Here's how the part is built. I have some questions about the finished solid (model axes, mm). Face numbers are marked on the shaded views. A direction names the side the tool comes from. Round coordinates to 2 decimals unless told otherwise and drop trailing zeros. Write each loop counter-clockwise with the first axis right and the second up, starting at its lowest first coordinate (ties: lowest second). Pieces come first, ordered by that corner, then holes. Notation, with made-up numbers: (21.25, 23) - (61.25, 23) arc R20 ccw to (61.25, 49) - close; hole circle Ø4 at (-6, -37). An arc over 180 degrees is marked (long way). Use one line per item in the form item = value. Start each with the question number.
1. Which directions (+Z, -Z, +X, -X, +Y, -Y) give clear straight access to the entire face, cutting with the end or side of a thin tool? Please do the marked faces 4, 5 and 6.
2. If I drill on line 1 along X through (y, z) = (29, 0); line 2 along X through (y, z) = (11.5, 0); line 3 along Y through (x, z) = (6, -18), over which ranges is the centre line in solid material (lowest first)?
3. We'd pull the mould along X, two halves only. Please class the marked faces 1, 2 and 3: +X half, -X half, draft (parallel to the pull), parting line (faces both ways), or undercut.
4. I want a section at D-D, the plane x = -38. List the corners of the cut face in (y, z) for me.
5. Will these pins go through, and if not, where does the flat tip stop? pin 1 (2 mm diameter, centred on x = -24.5, z = 5.5, fed in from -Y); pin 2 (12 mm diameter, centred on x = 18.5, z = -4, fed in from +Y); pin 3 (12 mm diameter, centred on y = 16.5, z = 0.5, fed in from -X); pin 4 (7.5 mm diameter, centred on y = 27, z = -1, fed in from +X).
6. I want a section at A-A, the plane z = 0. List the corners of the cut face in (x, y) for me.
7. I want a section at C-C, the plane y = 32. List the corners of the cut face in (x, z) for me.
8. I want a section at B-B, the plane x = -26.5. List the corners of the cut face in (y, z) for me.
```python
from build123d import *

# Parameters (mm, degrees)
SKETCH1_R           = 10
BOSS_EXTRUDE1_DEPTH = 10
SKETCH2_R           = 10
BOSS_EXTRUDE2_DEPTH = 30
SKETCH1_3_R         = 10
SKETCH1_3_R_2       = 8.299382461
BOSS_EXTRUDE3_DEPTH = 15
FILLET1_R           = 2
FILLET2_R           = 5


with BuildPart() as part:
    # Sketch1 → Boss-Extrude1 (new body)
    with BuildSketch(Plane(origin=(0, 0, 0), x_dir=(1, 0, 0), z_dir=(0, 1, 0))):
        with BuildLine():
            Line((-30, 20), (30, 20))
            ThreePointArc((30, 20), (50, 0), (30, -20))
            Line((30, -20), (-30, -20))
            ThreePointArc((-30, -20), (-50, 0), (-30, 20))
        make_face()
        with Locations(Location((-30, 0, 0), (0, 0, 270))):
            Circle(SKETCH1_R, mode=Mode.SUBTRACT)
        with Locations(Location((30, 0, 0), (0, 0, 270))):
            Circle(SKETCH1_R, mode=Mode.SUBTRACT)
    extrude(amount=BOSS_EXTRUDE1_DEPTH)

    # Sketch2 → Boss-Extrude2 (add)
    with BuildSketch(Plane(origin=(0, 10, 0), x_dir=(1, 0, 0), z_dir=(0, 1, 0))):
        with BuildLine():
            Line((-10, -20), (-30, -20))
            ThreePointArc((-30, -20), (-50, 0), (-30, 20))
            Line((-30, 20), (-10, 20))
            Line((-10, 20), (-10, -20))
        make_face()
        with Locations(Location((-30, 0, 0), (0, 0, 270))):
            Circle(SKETCH2_R, mode=Mode.SUBTRACT)
    extrude(amount=BOSS_EXTRUDE2_DEPTH)

    # Sketch1_3 → Boss-Extrude3 (add)
    with BuildSketch(Plane(origin=(0, 0, 0), x_dir=(1, 0, 0), z_dir=(0, 1, 0))):
        with Locations(Location((30, 0, 0), (0, 0, 270))):
            Circle(SKETCH1_3_R)
        with Locations(Location((30, 0, 0), (0, 0, 270))):
            Circle(SKETCH1_3_R_2, mode=Mode.SUBTRACT)
    extrude(amount=BOSS_EXTRUDE3_DEPTH)

    # Fillet1
    fillet1_edges = [part.edges().sort_by_distance(p)[0] for p in [
        (30, 10, -10),
    ]]
    fillet(fillet1_edges, radius=FILLET1_R)

    # Fillet2
    fillet2_edges = [part.edges().sort_by_distance(p)[0] for p in [
        (-10, 10, 0),
    ]]
    fillet(fillet2_edges, radius=FILLET2_R)


solid = part.part
```
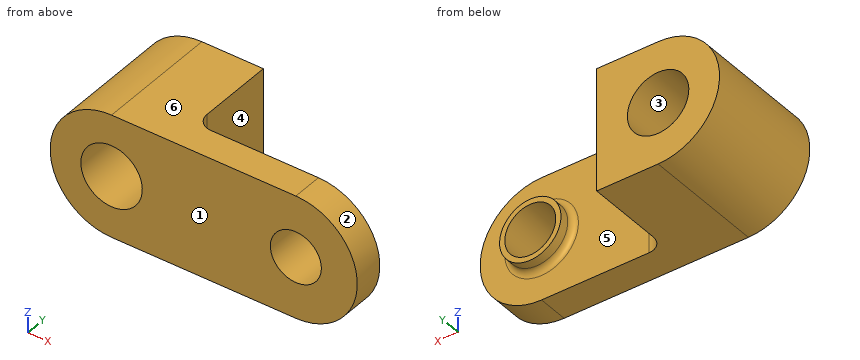
Model answer:
q1.face_4 = +Z, -Z, +X, +Y
q1.face_5 = +Y
q1.face_6 = +Z, +X, -X, +Y, -Y
q2.line_1 = -50 to -40, -20 to -10
q2.line_2 = -50 to -40, -20 to -8.57, 19.94 to 21.7, 38.3 to 40.06
q2.line_3 = 0 to 10
q3.face_1 = draft
q3.face_2 = +X half
q3.face_3 = undercut
q4.outline = (0, -18.33) - (40, -18.33) - (40, -6) - (0, -6) - close; (0, 6) - (40, 6) - (40, 18.33) - (0, 18.33) - close
q5.pin_1 = through
q5.pin_2 = 15
q5.pin_3 = -50
q5.pin_4 = -10
q6.outline = (-50, 0) - (-40, 0) - (-40, 40) - (-50, 40) - close; (-20, 0) - (21.7, 0) - (21.7, 15) - (20, 15) - (20, 12) arc R2 cw to (18, 10) - (-5, 10) arc R5 cw to (-10, 15) - (-10, 40) - (-20, 40) - close; (38.3, 0) - (50, 0) - (50, 10) - (42, 10) arc R2 cw to (40, 12) - (40, 15) - (38.3, 15) - close
q7.outline = (-30, -20) - (-10, -20) - (-10, 20) - (-30, 20) arc R20 ccw to start; hole circle Ø20 at (-30, 0)
q8.outline = (0, -20) - (40, -20) - (40, -9.37) - (0, -9.37) - close; (0, 9.37) - (40, 9.37) - (40, 20) - (0, 20) - close
